The listing builds one solid part. Answer for the finished solid, in the listing's coordinates (mm). Face numbers are marked on the shaded views. A direction names the side the tool comes from. Give positions to 0.01 mm unless a question says otherwise; leave off trailing zeros. Order: outer loops, then holes, each group sorted by start corner. A loop starts at its lowest first (then second) coordinate and runs counter-clockwise, first axis right, second up. Notation, with made-up numbers: (77, 47) - (135, 47) arc R13 ccw to (135, 62) - close; hole circle Ø8 at (69.5, -0.5). An arc over 180 degrees is marked (long way). Answer as a JSON object with one key per item and string values. Group by question number.
Q1. A cutting plane is placed at D-D, the plane z = 9. Give the vertices of the cut face in (x, y), and give its area (3 significant figures).
Q2. Given pin 1 (5 mm diameter, centred on x = 143, z = 49.1, fed in from -Y); pin 2 (2 mm diameter, centred on x = 76.5, z = 7, fed in from +Y); pin 3 (3.5 mm diameter, centred on x = 143, z = 5, fed in from -Y), each flat-ended and moving along its own axis, determine where each tip first touches the part or whether it passes through.
Q3. The mould has two halves that part along X. Classify the marked faces 1, 2, 3 and 4: released by +X, released by -X, zero draft, split by the parting line, or undercut.
Q4. For the marked faces 5, 6 and 7, determine the directions among +Z, -Z, +X, -X, +Y, -Y from which every point of the face is accessible in a straight line to the end or side of a thin tool.
Q5. A cutting plane is placed at A-A, the plane x = 24. Give the vertices of the cut face in (y, z).
Q6. A cutting plane is placed at C-C, the plane x = 110. Give the vertices of the cut face in (y, z).
Q7. Consider line 1 (Z direction, x = 55, y = -7.25); line 2 (Z direction, x = 24, y = -8.1); line 3 (Z direction, x = 100, y = -8.1). Determine where each line is inside the solid, lowest interval first.
Q8. A cutting plane is placed at B-B, the plane z = 40. Give the vertices of the cut face in (x, y).
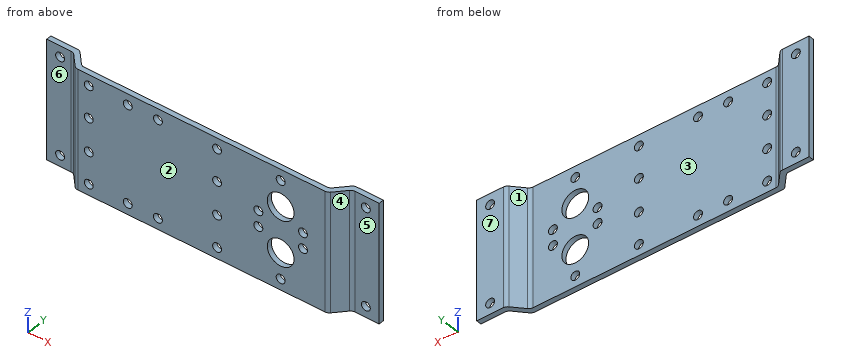
from build123d import *

# Parameters (mm, degrees)
BOSS_EXTRU_1_DEPTH      = 54.1
ESQUISSE2_R             = 2
ESQUISSE2_R_2           = 6
ENL_V_MAT_EXTRU_1_DEPTH = 9.8


with BuildPart() as part:
    # Esquisse1 → Boss.-Extru.1 (new body)
    with BuildSketch(Plane.XY):
        with BuildLine():
            Line((0, 0), (11.905421921, 0))
            ThreePointArc((11.905421921, 0), (12.908105659, -0.209885304), (13.742430532, -0.804299743))
            Line((13.742430532, -0.804299743), (18.257569468, -5.695700257))
            ThreePointArc((18.257569468, -5.695700257), (19.091894341, -6.290114696), (20.094578079, -6.5))
            Line((20.094578079, -6.5), (128.905421921, -6.5))
            ThreePointArc((128.905421921, -6.5), (129.908105659, -6.290114696), (130.742430532, -5.695700257))
            Line((130.742430532, -5.695700257), (135.257569468, -0.804299743))
            ThreePointArc((135.257569468, -0.804299743), (136.091894341, -0.209885304), (137.094578079, 0))
            Line((137.094578079, 0), (149, 0))
            Line((149, 0), (149, -2.3))
            Line((149, -2.3), (138.101589912, -2.3))
            ThreePointArc((138.101589912, -2.3), (137.098906174, -2.509885304), (136.264581301, -3.104299743))
            Line((136.264581301, -3.104299743), (131.749442365, -7.995700257))
            ThreePointArc((131.749442365, -7.995700257), (130.915117492, -8.590114696), (129.912433754, -8.8))
            Line((129.912433754, -8.8), (19.087566246, -8.8))
            ThreePointArc((19.087566246, -8.8), (18.084882508, -8.590114696), (17.250557635, -7.995700257))
            Line((17.250557635, -7.995700257), (12.735418699, -3.104299743))
            ThreePointArc((12.735418699, -3.104299743), (11.901093826, -2.509885304), (10.898410088, -2.3))
            Line((10.898410088, -2.3), (0, -2.3))
            Line((0, -2.3), (0, 0))
        make_face()
    extrude(amount=BOSS_EXTRU_1_DEPTH)

    # Esquisse2 → Enlèv. mat.-Extru.1 (cut, through all)
    with BuildSketch(Plane(origin=(0, 0, 0), x_dir=(1, 0, 0), z_dir=(0, 1, 0))):
        with Locations((6, -5)):
            Circle(ESQUISSE2_R)
        with Locations((24, -5)):
            Circle(ESQUISSE2_R)
        with Locations((41.5, -5)):
            Circle(ESQUISSE2_R)
        with Locations((55, -5)):
            Circle(ESQUISSE2_R)
        with Locations((81.5, -5)):
            Circle(ESQUISSE2_R)
        with Locations((110, -5)):
            Circle(ESQUISSE2_R)
        with Locations((143, -5)):
            Circle(ESQUISSE2_R)
        with Locations((120, -30.6)):
            Circle(ESQUISSE2_R)
        with Locations((100, -30.6)):
            Circle(ESQUISSE2_R)
        with Locations((110, -37.35)):
            Circle(ESQUISSE2_R_2)
        with Locations((81.5, -34.6)):
            Circle(ESQUISSE2_R)
        with Locations((24, -34.6)):
            Circle(ESQUISSE2_R)
        with Locations((143, -49.1)):
            Circle(ESQUISSE2_R)
        with Locations((110, -49.1)):
            Circle(ESQUISSE2_R)
        with Locations((24, -19.5)):
            Circle(ESQUISSE2_R)
        with Locations((81.5, -19.5)):
            Circle(ESQUISSE2_R)
        with Locations((110, -16.75)):
            Circle(ESQUISSE2_R_2)
        with Locations((120, -23.5)):
            Circle(ESQUISSE2_R)
        with Locations((100, -23.5)):
            Circle(ESQUISSE2_R)
        with Locations((81.5, -49.1)):
            Circle(ESQUISSE2_R)
        with Locations((55, -49.1)):
            Circle(ESQUISSE2_R)
        with Locations((41.5, -49.1)):
            Circle(ESQUISSE2_R)
        with Locations((24, -49.1)):
            Circle(ESQUISSE2_R)
        with Locations((6, -49.1)):
            Circle(ESQUISSE2_R)
    extrude(amount=-ENL_V_MAT_EXTRU_1_DEPTH, mode=Mode.SUBTRACT)


solid = part.part
Reply:
{
 "1": {"outline": "(0, -2.3) - (10.9, -2.3) arc R2.5 cw to (12.74, -3.1) - (17.25, -8) arc R2.5 ccw to (19.09, -8.8) - (129.91, -8.8) arc R2.5 ccw to (131.75, -8) - (136.26, -3.1) arc R2.5 cw to (138.1, -2.3) - (149, -2.3) - (149, 0) - (137.09, 0) arc R2.5 ccw to (135.26, -0.8) - (130.74, -5.7) arc R2.5 cw to (128.91, -6.5) - (20.09, -6.5) arc R2.5 cw to (18.26, -5.7) - (13.74, -0.8) arc R2.5 ccw to (11.91, 0) - (0, 0) - close", "area": "356 mm^2"},
 "2": {"pin 1": "stops at y = -2.3", "pin 2": "stops at y = -6.5", "pin 3": "passes through"},
 "3": {"face 1": "undercut", "face 2": "zero draft", "face 3": "undercut", "face 4": "released by +X"},
 "4": {"face 5": "+Z, -Z, +X, -Y", "face 6": "+Z, -Z, -X, -Y", "face 7": "+Z, -Z, +X, -X, +Y"},
 "5": {"outline": "(-8.8, 0) - (-6.5, 0) - (-6.5, 3) - (-8.8, 3) - close; (-8.8, 7) - (-6.5, 7) - (-6.5, 17.5) - (-8.8, 17.5) - close; (-8.8, 21.5) - (-6.5, 21.5) - (-6.5, 32.6) - (-8.8, 32.6) - close; (-8.8, 36.6) - (-6.5, 36.6) - (-6.5, 47.1) - (-8.8, 47.1) - close; (-8.8, 51.1) - (-6.5, 51.1) - (-6.5, 54.1) - (-8.8, 54.1) - close"},
 "6": {"outline": "(-8.8, 0) - (-6.5, 0) - (-6.5, 3) - (-8.8, 3) - close; (-8.8, 7) - (-6.5, 7) - (-6.5, 10.75) - (-8.8, 10.75) - close; (-8.8, 22.75) - (-6.5, 22.75) - (-6.5, 31.35) - (-8.8, 31.35) - close; (-8.8, 43.35) - (-6.5, 43.35) - (-6.5, 47.1) - (-8.8, 47.1) - close; (-8.8, 51.1) - (-6.5, 51.1) - (-6.5, 54.1) - (-8.8, 54.1) - close"},
 "7": {"line 1": "z = 0 to 3, 7 to 47.1, 51.1 to 54.1", "line 2": "z = 0 to 3, 7 to 17.5, 21.5 to 32.6, 36.6 to 47.1, 51.1 to 54.1", "line 3": "z = 0 to 21.5, 25.5 to 28.6, 32.6 to 54.1"},
 "8": {"outline": "(0, -2.3) - (10.9, -2.3) arc R2.5 cw to (12.74, -3.1) - (17.25, -8) arc R2.5 ccw to (19.09, -8.8) - (104.62, -8.8) - (104.62, -6.5) - (20.09, -6.5) arc R2.5 cw to (18.26, -5.7) - (13.74, -0.8) arc R2.5 ccw to (11.91, 0) - (0, 0) - close; (115.38, -8.8) - (129.91, -8.8) arc R2.5 ccw to (131.75, -8) - (136.26, -3.1) arc R2.5 cw to (138.1, -2.3) - (149, -2.3) - (149, 0) - (137.09, 0) arc R2.5 ccw to (135.26, -0.8) - (130.74, -5.7) arc R2.5 cw to (128.91, -6.5) - (115.38, -6.5) - close"}
}
